Autodesk Inventor part; units mm, degrees
ref_plane "YZ Plane" through (0, 0, 0) normal (1, 0, 0) x (0, 1, 0)
ref_plane "XZ Plane" through (0, 0, 0) normal (0, 1, 0) x (-1, 0, 0)
ref_plane "XY Plane" through (0, 0, 0) normal (0, 0, 1) x (1, 0, 0)
sketch "Sketch1" plane through (0, 0, 0) normal (0, 1, 0) x (-1, 0, 0)
  line L0 (0, 0) -> (81, 0)
  line L1 (81, 0) -> (81, -116)
  line L2 (81, -116) -> (0, -116)
  line L3 (0, -116) -> (0, 0)
  dimension "d0" = 81
  dimension "d1" = 116
extrude "Extrusion1" add sketch "Sketch1" along normal blind 3
sketch "Sketch2" plane through (0, 3, 0) normal (0, 1, 0) x (1, 0, 0)
  line L0 (0, 116) -> (-81, 116)
  line L1 (0, 0) -> (-81, 0)
  line L2 (-81, 0) -> (-81, 116)
  line L3 (-81, 116) -> (0, 116)
  line L4 (0, 116) -> (0, 0)
  line L5 (-3, 3) -> (-78, 3)
  line L6 (-78, 3) -> (-78, 113)
  line L7 (-78, 113) -> (-3, 113)
  line L8 (-3, 113) -> (-3, 3)
  dimension "d4" = 3
  dimension "d5" = 3
  dimension "d6" = 3
  dimension "d7" = 3
extrude "Extrusion2" add sketch "Sketch2" along normal blind 48
sketch "Sketch3" plane through (-81, 0, 0) normal (0, 0, 1) x (1, 0, 0)
  line L0 (0, 51) -> (81, 51)
  line L1 (0, 51) -> (81, 51)
  line L2 (81, 51) -> (81, 0)
  line L3 (81, 0) -> (0, 0)
  line L4 (0, 0) -> (0, 51)
extrude "Extrusion3" cut sketch "Sketch3" against normal up to surface (3 mm away)
sketch "Sketch4" plane through (0, 51, 0) normal (0, 1, 0) x (1, 0, 0)
  line L0 (-81, 116) -> (-81, 3)
  line L1 (0, 3) -> (0, 116)
  line L2 (-81, 116) -> (0, 116)
  line L3 (0, 116) -> (0, 113.2852)
  line L4 (0, 113.2852) -> (-81, 113.2852)
  line L5 (-81, 113.2852) -> (-81, 116)
  point P0 (0, 0)
  point P1 (0, 116)
extrude "Extrusion4" add sketch "Sketch4" along normal blind 6
sketch "Sketch5" plane through (0, 0, -116) normal (0, 0, -1) x (-1, 0, 0)
  line L0 (29.5, 55) -> (51.5, 55)
  line L1 (51.5, 55) -> (51.5, 51)
  line L2 (51.5, 51) -> (29.5, 51)
  line L3 (29.5, 51) -> (29.5, 55)
  line L4 (34.5, 30) -> (46.5, 30)
  line L5 (46.5, 30) -> (46.5, 18)
  line L6 (46.5, 18) -> (34.5, 18)
  line L7 (34.5, 18) -> (34.5, 30)
  line L8 (81, 0) -> (81, 57)
  line L9 (0, 0) -> (81, 0)
  line L10 (0, 57) -> (81, 57)
  point P0 (51.5, 53)
  dimension "d14" = 12
  dimension "d15" = 12
  dimension "d16" = 34.5
  dimension "d17" = 18
  dimension "d18" = 22
  dimension "d19" = 4
  dimension "d20" = 6
  dimension "d21" = 29.5
extrude "Extrusion5" cut sketch "Sketch5" against normal up to surface (3 mm away)
sketch "Sketch6" plane through (0, 0, -3) normal (1, 0, 0) x (0, 0, -1)
  line L0 (10, 31) -> (16, 31)
  line L1 (16, 31) -> (16, 16)
  line L2 (16, 16) -> (10, 16)
  line L3 (10, 16) -> (10, 31)
  line L4 (0, 51) -> (0, 0)
  line L5 (0, 0) -> (113, 0)
  point P0 (-3, 0)
  point P1 (13, 16)
  dimension "d24" = 6
  dimension "d25" = 15
  dimension "d26" = 10
  dimension "d27" = 16
extrude "Extrusion6" cut sketch "Sketch6" against normal up to surface (81 mm away)
properties part number "bin v1"
Work out the finished part from the listing and answer in its coordinate system (mm). A direction names the side the tool comes from. Give positions to 0.01 mm unless a question says otherwise; leave off trailing zeros. Loops run counter-clockwise (first coordinate to the right, second up) from the corner with the lowest first, then second, coordinate; pieces in that order, holes last. Notation, with made-up numbers: (29.25, 72) - (75.25, 72) arc R24 ccw to (75.25, 82) - close; hole circle Ø3 at (72.5, 14). An arc over 180 degrees is marked (long way). Answer in a Markdown table with one row per item.
(1) A tool of negligible diameter and unlimited length cuts with its end or side. For faces 5 (the face through (-51.5, 53, -115)), 6 (the face through (-1, 16, -16)), 7 (the face through (-78, 27, -57)), from which of +Z, -Z, +X, -X, +Y, -Y can it reach the whole face along a straight path? Write none if from no direction.
Results list:
| item | result |
|---|---|
| face 5 | +Z, -Z |
| face 6 | +X, -X |
| face 7 | +Z, +Y |
(2) Flat-ended cylindrical pins translate along their axes: pin 1 Ø0.9 at (x, z) = (-79.5, -14.5) entering from +Y; pin 2 Ø4 at (x, y) = (-29.5, 21) entering from +Z; pin 3 Ø4 at (x, z) = (-57.5, -24) entering from +Y. Find the tip coordinate at first contact, or state that the pin passes through.
Results list:
| item | result |
|---|---|
| pin 1 | stops at y = 51 |
| pin 2 | stops at z = -113 |
| pin 3 | stops at y = 3 |
(3) Section C-C (x = -19.5) is taken. Give the vertices of the cut face in (y, z), and give its area (3 significant figures).
Results list:
| item | result |
|---|---|
| outline | (0, -116) - (57, -116) - (57, -113.29) - (51, -113.29) - (51, -113) - (3, -113) - (3, -3) - (0, -3) - close |
| area | 499 mm² |
(4) Section A-A (y = 22) is taken. Give the vertices of the cut face in (x, z).
Results list:
| item | result |
|---|---|
| outline | (-81, -116) - (-46.5, -116) - (-46.5, -113) - (-78, -113) - (-78, -19) - (-81, -19) - close; (-81, -13) - (-78, -13) - (-78, -3) - (-81, -3) - close; (-34.5, -116) - (0, -116) - (0, -19) - (-3, -19) - (-3, -113) - (-34.5, -113) - close; (-3, -13) - (0, -13) - (0, -3) - (-3, -3) - close |
(5) For a pull along Z with two mould halves and no side action, classify faces 1 (the face through (-34.5, 24, -115)), 2 (the face through (-1, 31, -16)), 3 (the face through (-41, 34, -116)), 4 (the face through (-44, 1, -3)) as pulls with the +Z half, pulls with the -Z half, needs draft (parallel to the pull), parting line crosses it, or undercut.
Results list:
| item | result |
|---|---|
| face 1 | needs draft |
| face 2 | undercut |
| face 3 | pulls with the -Z half |
| face 4 | pulls with the +Z half |
(6) Consider L1, parallel to X at y = 24, z = -29; L2, parallel to Z at x = -44.5, y = 16.5; L3, parallel to Y at x = -24, z = -94.5. Determine where each line is inside the solid, lowest interval first. Write a range as [from, to].
Results list:
| item | result |
|---|---|
| L1 | x = [-81, -78], [-3, 0] |
| L2 | z = [-116, -113] |
| L3 | y = [0, 3] |
(7) Section B-B (z = -68) is taken. Give the vertices of the cut face in (x, y), and give its area (3 significant figures).
Results list:
| item | result |
|---|---|
| outline | (-81, 0) - (0, 0) - (0, 51) - (-3, 51) - (-3, 3) - (-78, 3) - (-78, 51) - (-81, 51) - close |
| area | 531 mm² |
